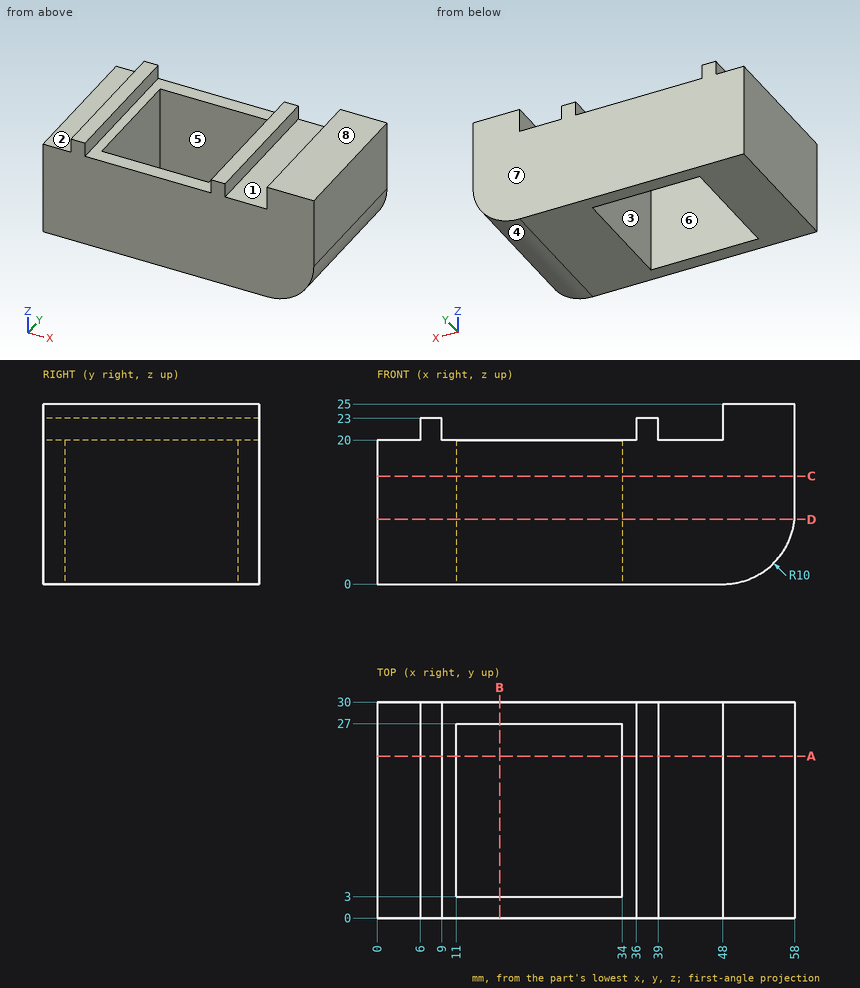
Drawing for the job (mm, zero at the part's lowest x, y, z). A direction names the side the tool comes from. Give positions to 0.01 mm unless a question says otherwise; leave off trailing zeros. Loops run counter-clockwise (first coordinate to the right, second up) from the corner with the lowest first, then second, coordinate; pieces in that order, holes last. Notation, with made-up numbers: M -5,84.25 L 39,84.25 A21 cw 39,88.25 Z; hole C -26,-37.5 d6. An arc over 180 degrees is marked long. One line per question, with ' | ' between items. Start each with the question number.
1. Saw through at B-B on x = 17. Give the cut face in (y, z), plus the area to 3 significant figures.
2. Saw through at A-A on y = 22.5. Give the cut face in (x, z), plus the area to 3 significant figures.
3. Saw through at D-D on z = 9. Give the cut face in (x, y), plus the area to 3 significant figures.
4. 3-axis set-ups, long thin cutter, end or side, ignore diameter. For the marked faces 1, 2, 3 and 4: which of +Z, -Z, +X, -X, +Y, -Y reach the whole face in a straight line?
5. Flat gauge pins, fed straight in: pin 1 (10 mm diameter, centred on y = 14, z = 5.5, fed in from +X); pin 2 (0.9 mm diameter, centred on y = 12.5, z = 21.5, fed in from -X); pin 3 (5 mm diameter, centred on x = 52, y = 25, fed in from -Z); pin 4 (6 mm diameter, centred on x = 34, y = 14, fed in from +Z). Where does each tip first touch, or does it go through?
6. Saw through at C-C on z = 15. Give the cut face in (x, y), plus the area to 3 significant figures.
7. Two-plate mould, pull along Y, no slides. Class the marked faces 5, 6, 7 and 8: pulls with the +Y half, pulls with the -Y half, needs draft (parallel to the pull), parting line crosses it, or undercut.
8. Probe L1, parallel to X at y = 12, z = 20.5; L2, parallel to Y at x = 12, z = 6.25; L3, parallel to X at y = 14.75, z = 17.5. List the from-to ranges inside material, lowest first. Write a range as from..to.
Result sheet:
1) outline: M 0,0 L 3,0 L 3,20 L 0,20 Z; M 27,0 L 30,0 L 30,20 L 27,20 Z | area: 120 mm^2
2) outline: M 0,0 L 11,0 L 11,20 L 9,20 L 9,23 L 6,23 L 6,20 L 0,20 Z; M 34,0 L 48,0 A10 ccw 58,10 L 58,25 L 48,25 L 48,20 L 39,20 L 39,23 L 36,23 L 36,20 L 34,20 Z | area: 747 mm^2
3) outline: M 0,0 L 57.95,0 L 57.95,30 L 0,30 Z; hole M 11,3 L 34,3 L 34,27 L 11,27 Z | area: 1,190 mm^2
4) face 1: +Z, +Y, -Y | face 2: +Z, -X, +Y, -Y | face 3: +Z, -Z | face 4: -Z, +X, +Y, -Y
5) pin 1: stops at x = 58 | pin 2: stops at x = 6 | pin 3: stops at z = 0.11 | pin 4: stops at z = 23
6) outline: M 0,0 L 58,0 L 58,30 L 0,30 Z; hole M 11,3 L 34,3 L 34,27 L 11,27 Z | area: 1,190 mm^2
7) face 5: undercut | face 6: undercut | face 7: pulls with the +Y half | face 8: needs draft
8) L1: x = 6..9, 36..39, 48..58 | L2: y = 0..3, 27..30 | L3: x = 0..11, 34..58
